from build123d import *

# Parameters (mm, degrees)
MODEL_R             = 3.5
EXTRUDE_1_DEPTH     = 40
SKETCH_3_W          = 37
SKETCH_3_H          = 37
CUT_EXTRUDE_1_DEPTH = 40
SKETCH_4_R          = 1.5
CUT_EXTRUDE_2_DEPTH = 40
SKETCH1_R           = 4
CUT_EXTRUDE1_DEPTH  = 10
SKETCH2_R           = 1.6
CUT_EXTRUDE2_DEPTH  = 10
SKETCH3_R           = 3
CUT_EXTRUDE3_DEPTH  = 1.5
SKETCH4_R           = 1.6
CUT_EXTRUDE4_DEPTH  = 10
SKETCH5_R           = 7.5
CUT_EXTRUDE5_DEPTH  = 10


with BuildPart() as part:
    # Model → 凸台-拉伸1 (new body)
    with BuildSketch(Plane.XY):
        with BuildLine():
            Line((2619.766714505, 1592.826425633), (2619.766714505, 1612.326425633))
            Line((2619.766714505, 1612.326425633), (2592.766714505, 1612.326425633))
            Line((2592.766714505, 1612.326425633), (2592.766714505, 1592.826425633))
            ThreePointArc((2592.766714505, 1592.826425633), (2606.266714505, 1579.326425633), (2619.766714505, 1592.826425633))
        make_face()
        with Locations((2606.266714505, 1592.826425633)):
            Circle(MODEL_R, mode=Mode.SUBTRACT)
    extrude(amount=EXTRUDE_1_DEPTH)

    # 草图3 → 切除-拉伸1 (cut)
    with BuildSketch(Plane(origin=(2619.766714505, 0, 0), x_dir=(0, 0, -1), z_dir=(1, 0, 0))):
        with Locations((-21.5, 1590.826425633)):
            Rectangle(SKETCH_3_W, SKETCH_3_H)
    extrude(amount=-CUT_EXTRUDE_1_DEPTH, mode=Mode.SUBTRACT)

    # 草图4 → 切除-拉伸2 (cut)
    with BuildSketch(Plane(origin=(0, 1612.326425633, 0), x_dir=(1, 0, 0), z_dir=(0, 1, 0))):
        with Locations(Location((2600.766714505, -32, 0), (0, 0, 270))):
            Circle(SKETCH_4_R)
        with Locations(Location((2611.766714505, -32, 0), (0, 0, 270))):
            Circle(SKETCH_4_R)
        with Locations(Location((2600.766714505, -12, 0), (0, 0, 270))):
            Circle(SKETCH_4_R)
        with Locations(Location((2611.766714505, -12, 0), (0, 0, 270))):
            Circle(SKETCH_4_R)
    extrude(amount=-CUT_EXTRUDE_2_DEPTH, mode=Mode.SUBTRACT)

    # Sketch1 → Cut-Extrude1 (cut)
    with BuildSketch(Plane(origin=(0, 0, 0), x_dir=(-1, 0, 0), z_dir=(0, 0, -1))):
        with Locations((-2606.266714505, 1592.826425633)):
            Circle(SKETCH1_R)
    extrude(amount=-CUT_EXTRUDE1_DEPTH, mode=Mode.SUBTRACT)

    # Sketch2 → Cut-Extrude2 (cut)
    with BuildSketch(Plane(origin=(0, 0, 0), x_dir=(-1, 0, 0), z_dir=(0, 0, -1))):
        with Locations((-2614.766714505, 1592.826425633)):
            Circle(SKETCH2_R)
        with Locations(Location((-2597.766714505, 1592.826425633, 0), (0, 0, 90))):
            Circle(SKETCH2_R)
    extrude(amount=-CUT_EXTRUDE2_DEPTH, mode=Mode.SUBTRACT)

    # Sketch3 → Cut-Extrude3 (cut)
    with BuildSketch(Plane(origin=(0, 0, 0), x_dir=(-1, 0, 0), z_dir=(0, 0, -1))):
        with Locations((-2597.766714505, 1592.826425633)):
            Circle(SKETCH3_R)
        with Locations((-2614.766714505, 1592.826425633)):
            Circle(SKETCH3_R)
    extrude(amount=-CUT_EXTRUDE3_DEPTH, mode=Mode.SUBTRACT)

    # Sketch4 → Cut-Extrude4 (cut)
    with BuildSketch(Plane(origin=(0, 1612.326425633, 0), x_dir=(1, 0, 0), z_dir=(0, 1, 0))):
        with Locations(Location((2600.766714505, -12, 0), (0, 0, 270))):
            Circle(SKETCH4_R)
        with Locations(Location((2611.766714505, -12, 0), (0, 0, 270))):
            Circle(SKETCH4_R)
        with Locations(Location((2600.766714505, -32, 0), (0, 0, 270))):
            Circle(SKETCH4_R)
        with Locations(Location((2611.766714505, -32, 0), (0, 0, 270))):
            Circle(SKETCH4_R)
    extrude(amount=-CUT_EXTRUDE4_DEPTH, mode=Mode.SUBTRACT)

    # Sketch5 → Cut-Extrude5 (cut)
    with BuildSketch(Plane(origin=(0, 1612.326425633, 0), x_dir=(1, 0, 0), z_dir=(0, 1, 0))):
        with Locations(Location((2606.266714505, -22, 0), (0, 0, 270))):
            Circle(SKETCH5_R)
    extrude(amount=-CUT_EXTRUDE5_DEPTH, mode=Mode.SUBTRACT)


solid = part.part
Could you check a few things on this model? Use its own coordinates, in mm. A direction names the side the tool comes from. Coordinates: 2 decimals unless noted, no trailing zeros. Order: outer loops, then holes, each group sorted by start corner. A loop starts at its lowest first (then second) coordinate and runs counter-clockwise, first axis right, second up. Notation, with made-up numbers: (42, 40) -> (87, 40) arc R15 ccw to (87, 51) -> close; hole circle Ø9 at (-4, -15). An arc over 180 degrees is marked (long way). One line per item, written item: value. Start each with the question number.
1) Imagine slicing it at B-B on z = 32. List the corners of the cut face in (x, y) for me.
2) If I drill on L1, parallel to X at y = 1610, z = 32; L2, parallel to X at y = 1610.85, z = 22; L3, parallel to Z at x = 2600.25, y = 1600, over which ranges is the centre line in solid material (lowest first)? Write a range as [from, to].
3) Imagine slicing it at D-D on x = 2596.75. List the corners of the cut face in (y, z) for me.
4) We'd pull the mould along X, two halves only. Please class faces 4 (the cylindrical face through (2602.45, 1594.03, 1.48)), 5 (the flat face through (2619.767, 1610, 14)), 6 (the flat face through (2606, 1611, 40)), 7 (the cylindrical face through (2605.97, 1579.33, 1.48)): +X half, -X half, draft (parallel to the pull), parting line (faces both ways), or undercut.
5) Imagine slicing it at C-C on y = 1590.5. List the corners of the cut face in (x, z) for me, plus the area to 3 significant figures.
6) Which directions (+Z, -Z, +X, -X, +Y, -Y) give clear straight access to the entire face, cutting with the end or side of a thin tool? Please do faces 1 (the cylindrical face through (2613.116, 1610.847, 12.86)), 2 (the cylindrical face through (2596.154, 1595.356, 0.74)), 3 (the flat face through (2606, 1609.326, 30)).
7) I'm going to push flat-ended pins straight in: pin 1 (9 mm diameter, centred on x = 2606.27, y = 1592.83, fed in from +Z); pin 2 (3.5 mm diameter, centred on x = 2600.77, z = 32, fed in from -Y); pin 3 (1.8 mm diameter, centred on x = 2597.5, y = 1592, fed in from -Z); pin 4 (13.5 mm diameter, centred on x = 2606.27, z = 22, fed in from -Y). Where does each tip first touch, or does it pass through?
8) Imagine slicing it at A-A on z = 22. List the corners of the cut face in (x, y) for me, plus the area to 3 significant figures.
Answer list:
1. outline: (2592.77, 1609.33) -> (2599.17, 1609.33) -> (2599.17, 1612.33) -> (2592.77, 1612.33) -> close; (2602.37, 1609.33) -> (2610.17, 1609.33) -> (2610.17, 1612.33) -> (2602.37, 1612.33) -> close; (2613.37, 1609.33) -> (2619.77, 1609.33) -> (2619.77, 1612.33) -> (2613.37, 1612.33) -> close
2. L1: x = [2592.77, 2599.17], [2602.37, 2610.17], [2613.37, 2619.77]
2. L2: x = [2592.77, 2598.77], [2613.77, 2619.77]
2. L3: z = [0, 3]
3. outline: (1583.25, 0) -> (1590, 0) -> (1590, 1.5) -> (1591.59, 1.5) -> (1591.59, 3) -> (1583.25, 3) -> close; (1594.06, 1.5) -> (1595.65, 1.5) -> (1595.65, 0) -> (1612.33, 0) -> (1612.33, 40) -> (1609.33, 40) -> (1609.33, 3) -> (1594.06, 3) -> close
4. face 4: undercut
4. face 5: +X half
4. face 6: draft
4. face 7: parting line
5. outline: (2592.97, 0) -> (2595.87, 0) -> (2595.87, 1.5) -> (2599.66, 1.5) -> (2599.66, 0) -> (2603.01, 0) -> (2603.01, 3) -> (2592.97, 3) -> close; (2609.52, 0) -> (2612.87, 0) -> (2612.87, 1.5) -> (2616.66, 1.5) -> (2616.66, 0) -> (2619.56, 0) -> (2619.56, 3) -> (2609.52, 3) -> close
5. area: 48.9 mm2
6. face 1: +Y, -Y
6. face 2: -Z
6. face 3: +Z, +X, -X, -Y
7. pin 1: stops at z = 3
7. pin 2: stops at y = 1609.33
7. pin 3: stops at z = 1.5
7. pin 4: passes through
8. outline: (2592.77, 1609.33) -> (2598.77, 1609.33) -> (2598.77, 1612.33) -> (2592.77, 1612.33) -> close; (2613.77, 1609.33) -> (2619.77, 1609.33) -> (2619.77, 1612.33) -> (2613.77, 1612.33) -> close
8. area: 36.0 mm2
